from build123d import *

# Parameters (mm, degrees)
BOSS_EXTRUDE1_DEPTH    = 17.539999972
F_10_CLEARANCE_HOLE1_D = 5.1054
SKETCH3_W              = 150
SKETCH3_H              = 75
CUT_EXTRUDE1_DEPTH     = 14.999999972
SKETCH4_W              = 155.08
SKETCH4_H              = 71.825
CUT_EXTRUDE2_DEPTH     = 13.412499972
CUT_EXTRUDE3_DEPTH     = 7.5
FILLET2_R              = 5.9125
FILLET1_R              = 7.5
FILLET3_R              = 3.175


with BuildPart() as part:
    # Sketch1 → Boss-Extrude1 (new body)
    with BuildSketch(Plane(origin=(0, 0, 0), x_dir=(1, 0, 0), z_dir=(0, 1, 0))):
        with BuildLine():
            Line((77.54, -40.04), (77.54, 40.04))
            Line((77.54, 40.04), (77.54, 46.39))
            ThreePointArc((77.54, 46.39), (71.19, 52.74), (64.84, 46.39))
            Line((64.84, 46.39), (64.84, 40.04))
            Line((64.84, 40.04), (-64.84, 40.04))
            Line((-64.84, 40.04), (-64.84, 46.39))
            ThreePointArc((-64.84, 46.39), (-71.19, 52.74), (-77.54, 46.39))
            Line((-77.54, 46.39), (-77.54, 40.04))
            Line((-77.54, 40.04), (-77.54, -40.04))
            Line((-77.54, -40.04), (-77.54, -46.39))
            ThreePointArc((-77.54, -46.39), (-71.19, -52.74), (-64.84, -46.39))
            Line((-64.84, -46.39), (-64.84, -40.04))
            Line((-64.84, -40.04), (64.84, -40.04))
            Line((64.84, -40.04), (64.84, -46.39))
            ThreePointArc((64.84, -46.39), (71.19, -52.74), (77.54, -46.39))
            Line((77.54, -46.39), (77.54, -40.04))
        make_face()
    extrude(amount=BOSS_EXTRUDE1_DEPTH)

    # #10 Clearance Hole1 (through all)
    with Locations(Plane(origin=(0, 17.539999972, 0), x_dir=(1, 0, 0), z_dir=(0, 1, 0))):
        with Locations((-71.19, 46.39), (71.19, 46.39), (71.19, -46.39), (-71.19, -46.39)):
            Hole(F_10_CLEARANCE_HOLE1_D / 2)

    # Sketch3 → Cut-Extrude1 (cut)
    with BuildSketch(Plane(origin=(0, 17.539999972, 0), x_dir=(1, 0, 0), z_dir=(0, 1, 0))):
        Rectangle(SKETCH3_W, SKETCH3_H)
    extrude(amount=-CUT_EXTRUDE1_DEPTH, mode=Mode.SUBTRACT)

    # Sketch4 → Cut-Extrude2 (cut)
    with BuildSketch(Plane(origin=(0, 17.539999972, 0), x_dir=(1, 0, 0), z_dir=(0, 1, 0))):
        Rectangle(SKETCH4_W, SKETCH4_H)
    extrude(amount=-CUT_EXTRUDE2_DEPTH, mode=Mode.SUBTRACT)

    # Sketch8 → Cut-Extrude3 (cut)
    with BuildSketch(Plane(origin=(0, 17.539999972, 0), x_dir=(1, 0, 0), z_dir=(0, 1, 0))):
        Polygon((-77.54, 37.5), (-64.84, 37.5), (-64.84, 40.04), (64.84, 40.04), (64.84, 37.5), (77.54, 37.5), (77.54, -37.5), (64.84, -37.5), (64.84, -40.04), (-64.84, -40.04), (-64.84, -37.5), (-77.54, -37.5), align=None)
    extrude(amount=-CUT_EXTRUDE3_DEPTH, mode=Mode.SUBTRACT)

    # Fillet2
    fillet2_edges = [part.edges().sort_by_distance(p)[0] for p in [
        (-76.27, 4.1275, -35.9125),
        (-76.27, 4.1275, 35.9125),
        (76.27, 4.1275, 35.9125),
        (76.27, 4.1275, -35.9125),
    ]]
    fillet(fillet2_edges, radius=FILLET2_R - 0.0001)  # a hair under: the kernel refuses the full size

    # Fillet1
    fillet1_edges = [part.edges().sort_by_distance(p)[0] for p in [
        (0, 2.54, 37.5),
        (0, 2.54, -37.5),
    ]]
    fillet(fillet1_edges, radius=FILLET1_R - 0.0001)  # a hair under: the kernel refuses the full size

    # Fillet3
    fillet3_edges = [part.edges().sort_by_distance(p)[0] for p in [
        (64.84, 5.019999986, 40.04),
        (-64.84, 5.019999986, 40.04),
        (-64.84, 5.019999986, -40.04),
        (64.84, 5.019999986, -40.04),
    ]]
    fillet(fillet3_edges, radius=FILLET3_R)


solid = part.part
Check sheet for the modelled part. Datum: model origin and axes. Units: mm. A direction names the side the tool comes from. Round coordinates to 2 decimals unless told otherwise and drop trailing zeros. Loops run counter-clockwise (first coordinate to the right, second up) from the corner with the lowest first, then second, coordinate; pieces in that order, holes last.
1. Scan lines: probe 1 along Z at (x, y) = (71.19, 10); probe 2 along X at (y, z) = (7.25, -46.39); probe 3 along Z at (x, y) = (71.19, 4.25). Record each from-to range of solid material in increasing order.
2. Sectioned sample at B-B on x = -71.19. Record the boundary of the cut face in (y, z), and give its area (3 significant figures).
3. Sectioned sample at D-D on z = -26.5. Record the boundary of the cut face in (x, y), and give its area (3 significant figures).
4. Mould release check, pull along X, two halves, no side actions. Record for faces 5 (the cylindrical face through (-71.05, 8.65, -52.74)), 6 (the flat face through (77.54, 3, 1)), 7 (the flat face through (-77.54, 3, -1)): released by +X, released by -X, zero draft, split by the parting line, or undercut.
5. Set-up check for faces 1 (the flat face through (64.84, 11, -43)), 2 (the cylindrical face through (63.93, 5.09, 40.99)), 3 (the flat face through (-64.84, 11, 43)), 4 (the cylindrical face through (1.05, 4.795, 35.361)): record each of +Z, -Z, +X, -X, +Y, -Y from which the full face is reachable in a straight line by a thin tool's end or side.
6. Sectioned sample at C-C on y = 7.75. Give the number of separate pieces and of enclosed holes in the cut face, and give its area (3 significant figures).
7. Sectioned sample at A-A on y = 15.25. Record the boundary of the cut face in (x, z), and give its area (3 significant figures).
8. Gauge pin test, flat ends, axial feed: pin 1 Ø8 at (x, y) = (35.5, 15.5) entering from +Z; pin 2 Ø1 at (x, z) = (14, -15.5) entering from +Y; pin 3 Ø1.3 at (x, z) = (-76.5, 12) entering from +Y; pin 4 Ø4.5 at (x, z) = (31, 39.5) entering from +Y. Record the tip position at first contact, or that the pin passes through.
Recorded:
1. probe 1: z = -52.74 to -48.94, -43.84 to -37.5, 37.5 to 43.84, 48.94 to 52.74
1. probe 2: x = -77.54 to -73.74, -68.64 to -64.84, 64.84 to 68.64, 73.74 to 77.54
1. probe 3: z = -52.74 to -48.94, -43.84 to -34.77, 34.77 to 43.84, 48.94 to 52.74
2. outline: (0, -52.74) - (17.54, -52.74) - (17.54, -48.94) - (0, -48.94) - close; (0, -43.84) - (17.54, -43.84) - (17.54, -37.5) - (10.04, -37.5) arc R7.5 cw to (2.54, -30) - (2.54, 30) arc R7.5 cw to (10.04, 37.5) - (17.54, 37.5) - (17.54, 43.84) - (0, 43.84) - close; (0, 48.94) - (17.54, 48.94) - (17.54, 52.74) - (0, 52.74) - close
2. area: 570 mm2
3. outline: (-77.54, 0) - (77.54, 0) - (77.54, 4.13) - (75, 4.13) - (75, 2.54) - (-75, 2.54) - (-75, 4.13) - (-77.54, 4.13) - close
3. area: 402 mm2
4. face 5: undercut
4. face 6: released by +X
4. face 7: released by -X
5. face 1: -Z, +Y
5. face 2: +Z, +Y, -Y
5. face 3: +Z, +Y
5. face 4: +Y
6. separate pieces: 2
6. enclosed holes: 4
6. area: 1,420 mm2
7. outline: (-77.54, -46.39) arc R6.35 ccw to (-64.84, -46.39) - (-64.84, -37.5) - (-77.54, -37.5) - close; (-77.54, 37.5) - (-64.84, 37.5) - (-64.84, 46.39) arc R6.35 ccw to (-77.54, 46.39) - close; (64.84, -46.39) arc R6.35 ccw to (77.54, -46.39) - (77.54, -37.5) - (64.84, -37.5) - close; (64.84, 37.5) - (77.54, 37.5) - (77.54, 46.39) arc R6.35 ccw to (64.84, 46.39) - close; hole circle Ø5.11 at (-71.19, -46.39); hole circle Ø5.11 at (-71.19, 46.39); hole circle Ø5.11 at (71.19, -46.39); hole circle Ø5.11 at (71.19, 46.39)
7. area: 623 mm2
8. pin 1: passes through
8. pin 2: stops at y = 2.54
8. pin 3: stops at y = 4.13
8. pin 4: stops at y = 10.04
